```python
from build123d import *

# Parameters (mm, degrees)
SKETCH1_W           = 61.4
SKETCH1_H           = 66.34
SKETCH1_R           = 1.55
BOSS_EXTRUDE1_DEPTH = 5


with BuildPart() as part:
    # Sketch1 → Boss-Extrude1 (new body)
    with BuildSketch(Plane(origin=(0, 0, 0), x_dir=(1, 0, 0), z_dir=(0, 1, 0))):
        with Locations((9.719215892, -3.98392863)):
            Rectangle(SKETCH1_W, SKETCH1_H)
        with Locations(Location((-18.480784108, 26.68607137, 0), (0, 0, 270))):
            Circle(SKETCH1_R, mode=Mode.SUBTRACT)
        with Locations(Location((37.919215892, 26.68607137, 0), (0, 0, 90))):
            Circle(SKETCH1_R, mode=Mode.SUBTRACT)
        with Locations(Location((37.919215892, -34.65392863, 0), (0, 0, 270))):
            Circle(SKETCH1_R, mode=Mode.SUBTRACT)
        with Locations(Location((-18.480784108, -34.65392863, 0), (0, 0, 90))):
            Circle(SKETCH1_R, mode=Mode.SUBTRACT)
        with BuildLine():
            Line((-12.755784108, -30.33892863), (32.194215892, -30.33892863))
            ThreePointArc((32.194215892, -30.33892863), (34.315536235, -29.460248974), (35.194215892, -27.33892863))
            Line((35.194215892, -27.33892863), (35.194215892, 19.37107137))
            ThreePointArc((35.194215892, 19.37107137), (34.315536235, 21.492391714), (32.194215892, 22.37107137))
            Line((32.194215892, 22.37107137), (-12.755784108, 22.37107137))
            ThreePointArc((-12.755784108, 22.37107137), (-14.877104452, 21.492391714), (-15.755784108, 19.37107137))
            Line((-15.755784108, 19.37107137), (-15.755784108, -27.33892863))
            ThreePointArc((-15.755784108, -27.33892863), (-14.877104452, -29.460248974), (-12.755784108, -30.33892863))
        make_face(mode=Mode.SUBTRACT)
    extrude(amount=BOSS_EXTRUDE1_DEPTH)


solid = part.part
```
Input: part model. Units: mm. Frame: model coordinates. A direction names the side the tool comes from. Coordinates: 2 decimals unless noted, no trailing zeros. Order: outer loops, then holes, each group sorted by start corner. A loop starts at its lowest first (then second) coordinate and runs counter-clockwise, first axis right, second up. Notation, with made-up numbers: (13, 5.25) - (67, 5.25) arc R19 ccw to (67, 35.25) - close; hole circle Ø5 at (-18, -30). An arc over 180 degrees is marked (long way). Put each result on its own line as item: value.
1. Draft query along X for faces 1 (the face through (-18, 0, 4)), 2 (the face through (39.432, 2.465, -26.35)), 3 (the face through (-20.981, 2, 4)). Return one class per face: pulls with the +X half, pulls with the -X half, needs draft (parallel to the pull), parting line crosses it, or undercut.
Report:
face 1: needs draft
face 2: undercut
face 3: pulls with the -X half
2. Reachability of faces 4 (the face through (34.292, 2.465, 29.483)), 5 (the face through (40.419, 2, 4)) from +Z, -Z, +X, -X, +Y, -Y: full face, straight path, thin tool, end or side. Return the list, or none.
Report:
face 4: +Y, -Y
face 5: +Z, -Z, +X, +Y, -Y
3. Line query: line 1 along Z through (x, y) = (-5, 3.75); line 2 along X through (y, z) = (2.65, -5); line 3 along X through (y, z) = (2.3, 33.5). Output: solid intervals per line, ascending.
Report:
line 1: z = -29.19 to -22.37, 30.34 to 37.15
line 2: x = -20.98 to -15.76, 35.19 to 40.42
line 3: x = -20.98 to -19.52, -17.45 to 36.88, 38.95 to 40.42
4. Cut plane A-A on z = 5. Return the cut outline in (x, y).
Report:
outline: (-20.98, 0) - (-15.76, 0) - (-15.76, 5) - (-20.98, 5) - close; (35.19, 0) - (40.42, 0) - (40.42, 5) - (35.19, 5) - close
5. Cut plane C-C on y = 3.1. Return the cut outline in (x, z).
Report:
outline: (-20.98, -29.19) - (40.42, -29.19) - (40.42, 37.15) - (-20.98, 37.15) - close; hole circle Ø3.1 at (-18.48, -26.69); hole circle Ø3.1 at (-18.48, 34.65); hole (-15.76, -19.37) arc R3 ccw to (-12.76, -22.37) - (32.19, -22.37) arc R3 ccw to (35.19, -19.37) - (35.19, 27.34) arc R3 ccw to (32.19, 30.34) - (-12.76, 30.34) arc R3 ccw to (-15.76, 27.34) - close; hole circle Ø3.1 at (37.92, -26.69); hole circle Ø3.1 at (37.92, 34.65)
6. Contact query for a flat-ended pin moving along its axis: pin 1 Ø4 at (x, z) = (-18.48, -26.69) entering from -Y. Output: stop coordinate, or through.
Report:
pin 1: stops at y = 0
7. Cut plane B-B on x = -3.5. Return the cut outline in (y, z), then the cut area to 4 significant figures.
Report:
outline: (0, -29.19) - (5, -29.19) - (5, -22.37) - (0, -22.37) - close; (0, 30.34) - (5, 30.34) - (5, 37.15) - (0, 37.15) - close
area: 68.15 mm2
